from build123d import *
from OCP.BRepFilletAPI import BRepFilletAPI_MakeChamfer

# Parameters (mm, degrees)
SKETCH_47_W         = 56
SKETCH_47_H         = 48
EXTRUDE_4_DEPTH     = 43
CHAMFER_1_SIZE      = 10
CHAMFER_1_SIZE2     = 3.639702343
SHELL_1_T           = -3
CUT_EXTRUDE_3_REACH = 86.392
SKETCH_48_R         = 1
SKETCH_48_W         = 23.8
SKETCH_48_H         = 12.2
SKETCH_49_R         = 1.55
CUT_EXTRUDE_4_DEPTH = 71.263788682
CUT_EXTRUDE_5_REACH = 76.572
SKETCH_50_W         = 13
SKETCH_50_H         = 9
CUT_EXTRUDE_6_REACH = 76.572
SKETCH_51_W         = 10.719183514
SKETCH_51_H         = 21.879791556


with BuildPart() as part:
    # 草图47 → 凸台-拉伸4 (new body)
    with BuildSketch(Plane(origin=(0, 0, 0), x_dir=(1, 0, 0), z_dir=(0, 1, 0))):
        Rectangle(SKETCH_47_W, SKETCH_47_H)
    extrude(amount=EXTRUDE_4_DEPTH)

    # 倒角1: one chamfer whose edges measure the first distance from different faces: ONE call of the kernel's chamfer builder (chamfer() names one face for all edges)
    chamfer_1_edges_1 = [part.edges().sort_by_distance(p)[0] for p in [
        (28, 43, 0),
    ]]
    chamfer_1_side_1 = [part.faces().sort_by_distance(p)[0] for p in [
        (28, 21.5, 0),
    ]]
    chamfer_1_edges_2 = [part.edges().sort_by_distance(p)[0] for p in [
        (0, 43, -24),
    ]]
    chamfer_1_side_2 = [part.faces().sort_by_distance(p)[0] for p in [
        (0, 21.5, -24),
    ]]
    chamfer_1_edges_3 = [part.edges().sort_by_distance(p)[0] for p in [
        (-28, 43, 0),
    ]]
    chamfer_1_side_3 = [part.faces().sort_by_distance(p)[0] for p in [
        (-28, 21.5, 0),
    ]]
    chamfer_1_edges_4 = [part.edges().sort_by_distance(p)[0] for p in [
        (0, 43, 24),
    ]]
    chamfer_1_side_4 = [part.faces().sort_by_distance(p)[0] for p in [
        (0, 21.5, 24),
    ]]
    chamfer_1 = BRepFilletAPI_MakeChamfer(part.part.solid().wrapped)
    for e in chamfer_1_edges_1:
        chamfer_1.Add(CHAMFER_1_SIZE, CHAMFER_1_SIZE2, e.wrapped, chamfer_1_side_1[0].wrapped)  # the first distance lies on this face
    for e in chamfer_1_edges_2:
        chamfer_1.Add(CHAMFER_1_SIZE, CHAMFER_1_SIZE2, e.wrapped, chamfer_1_side_2[0].wrapped)  # the first distance lies on this face
    for e in chamfer_1_edges_3:
        chamfer_1.Add(CHAMFER_1_SIZE, CHAMFER_1_SIZE2, e.wrapped, chamfer_1_side_3[0].wrapped)  # the first distance lies on this face
    for e in chamfer_1_edges_4:
        chamfer_1.Add(CHAMFER_1_SIZE, CHAMFER_1_SIZE2, e.wrapped, chamfer_1_side_4[0].wrapped)  # the first distance lies on this face
    add(Compound.cast(chamfer_1.Shape()), mode=Mode.REPLACE)

    # 抽壳1
    shell_1_openings = [part.faces().sort_by_distance(p)[0] for p in [
        (0, 0, 0),
    ]]
    offset(amount=SHELL_1_T, openings=shell_1_openings, kind=Kind.INTERSECTION)

    # 草图48 → 切除-拉伸3 (cut, up to next)
    with BuildSketch(Plane(origin=(0, 43, -43), x_dir=(1, 0, 0), z_dir=(0, -1, 0)), mode=Mode.PRIVATE) as cut_extrude_3_sk1:
        with Locations(Location((-20.1, 43, 0), (0, 0, 90))):
            Circle(SKETCH_48_R)
    cut_extrude_3_tool1 = extrude(cut_extrude_3_sk1.sketch, amount=CUT_EXTRUDE_3_REACH, mode=Mode.PRIVATE) & part.part
    # 草图48 → 切除-拉伸3 (cut, up to next)
    with BuildSketch(Plane(origin=(0, 43, -43), x_dir=(1, 0, 0), z_dir=(0, -1, 0)), mode=Mode.PRIVATE) as cut_extrude_3_sk2:
        with Locations(Location((8.5, 43, 0), (0, 0, 90))):
            Circle(SKETCH_48_R)
    cut_extrude_3_tool2 = extrude(cut_extrude_3_sk2.sketch, amount=CUT_EXTRUDE_3_REACH, mode=Mode.PRIVATE) & part.part
    # 草图48 → 切除-拉伸3 (cut, up to next)
    with BuildSketch(Plane(origin=(0, 43, -43), x_dir=(1, 0, 0), z_dir=(0, -1, 0)), mode=Mode.PRIVATE) as cut_extrude_3_sk3:
        with Locations((-5.8, 43)):
            Rectangle(SKETCH_48_W, SKETCH_48_H)
    cut_extrude_3_tool3 = extrude(cut_extrude_3_sk3.sketch, amount=CUT_EXTRUDE_3_REACH, mode=Mode.PRIVATE) & part.part
    add(cut_extrude_3_tool1.solids().sort_by_distance((-20.1, 43, 0))[0], mode=Mode.SUBTRACT)
    add(cut_extrude_3_tool2.solids().sort_by_distance((8.5, 43, 0))[0], mode=Mode.SUBTRACT)
    add(cut_extrude_3_tool3.solids().sort_by_distance((-5.8, 43, 0))[0], mode=Mode.SUBTRACT)

    # 草图49 → 切除-拉伸4 (cut, through all)
    with BuildSketch(Plane(origin=(0, 0, -24), x_dir=(-1, 0, 0), z_dir=(0, 0, -1))):
        with Locations((0, 8)):
            Circle(SKETCH_49_R)
    extrude(amount=-CUT_EXTRUDE_4_DEPTH, mode=Mode.SUBTRACT)

    # 草图50 → 切除-拉伸5 (cut, up to next)
    with BuildSketch(Plane(origin=(28, 0, 0), x_dir=(0, 0, -1), z_dir=(1, 0, 0)), mode=Mode.PRIVATE) as cut_extrude_5_sk1:
        with Locations((0, 4.5)):
            Rectangle(SKETCH_50_W, SKETCH_50_H)
    cut_extrude_5_tool1 = extrude(cut_extrude_5_sk1.sketch, amount=-CUT_EXTRUDE_5_REACH, mode=Mode.PRIVATE) & part.part
    add(cut_extrude_5_tool1.solids().sort_by_distance((28, 4.5, 0))[0], mode=Mode.SUBTRACT)

    # 草图51 → 切除-拉伸6 (cut, up to next)
    with BuildSketch(Plane.ZY.offset(28), mode=Mode.PRIVATE) as cut_extrude_6_sk1:
        with Locations((0, 10.939895778)):
            Rectangle(SKETCH_51_W, SKETCH_51_H)
    cut_extrude_6_tool1 = extrude(cut_extrude_6_sk1.sketch, amount=-CUT_EXTRUDE_6_REACH, mode=Mode.PRIVATE) & part.part
    add(cut_extrude_6_tool1.solids().sort_by_distance((-28, 10.939896, 0))[0], mode=Mode.SUBTRACT)


solid = part.part
Part model, mm, in its own coordinate system. A direction names the side the tool comes from. Give positions to 0.01 mm unless a question says otherwise; leave off trailing zeros. Order: outer loops, then holes, each group sorted by start corner. A loop starts at its lowest first (then second) coordinate and runs counter-clockwise, first axis right, second up. Notation, with made-up numbers: (-21, 3) -> (38, 3) arc R13 ccw to (38, 13) -> close; hole circle Ø6 at (5.25, 22). An arc over 180 degrees is marked (long way). Use one line per item in the form item = value.
(1) Saw through at D-D (y = 21). Write the cut outline in (x, z), then the cut area to 3 significant figures.
Solution:
outline = (-28, -24) -> (28, -24) -> (28, 24) -> (-28, 24) -> (-28, 5.36) -> (-25, 5.36) -> (-25, 21) -> (25, 21) -> (25, -21) -> (-25, -21) -> (-25, -5.36) -> (-28, -5.36) -> close
area = 556 mm²
(2) Drill centre lines: line 1 (Z direction, x = -15, y = 14.5); line 2 (X direction, y = 41.7, z = 0); line 3 (X direction, y = 7, z = 17). Where is each one in solid material? Low to high. Write a range as from..to.
Solution:
line_1 = -24..-21, 21..24
line_2 = -24.83..-21.1, -19.1..-17.7, 6.1..7.5, 9.5..24.83
line_3 = -28..-25, 25..28
(3) Saw through at C-C (z = 0). Write the cut outline in (x, y), then the cut area to 3 significant figures.
Solution:
outline = (-28, 21.88) -> (-25, 21.88) -> (-25, 32.47) -> (-22.26, 40) -> (-21.1, 40) -> (-21.1, 43) -> (-24.36, 43) -> (-28, 33) -> close; (-19.1, 40) -> (-17.7, 40) -> (-17.7, 43) -> (-19.1, 43) -> close; (6.1, 40) -> (7.5, 40) -> (7.5, 43) -> (6.1, 43) -> close; (9.5, 40) -> (22.26, 40) -> (25, 32.47) -> (25, 9) -> (28, 9) -> (28, 33) -> (24.36, 43) -> (9.5, 43) -> close
area = 216 mm²
(4) Flat gauge pins, fed straight in: P1, Ø6, axis at y = 34, z = 9, coming from the -X side; P2, Ø4, axis at x = -12, y = 37.5, coming from the -Z side; P3, Ø0.9, axis at x = -3.5, y = 41.5, coming from the -Z side; P4, Ø1.9, axis at x = 0, y = 8, coming from the -Z side. Where does each tip first touch, or does it go through?
Solution:
P1 = -28
P2 = -23.09
P3 = -21.07
P4 = through
(5) Tool access for faces 5 (the face through (6.1, 42, 0)), 6 (the face through (0, 16, -21)), 7 (the face through (-27, 11, 5.36)): list every direction of +Z, -Z, +X, -X, +Y, -Y with a clear straight run to the whole face (end or side of a thin tool).
Solution:
face_5 = +Y, -Y
face_6 = -Y
face_7 = -X, -Y
(6) Pull direction X, two halves, no side cores. Call faces 1 (the face through (-0.715, 6.625, -22.521)), 2 (the face through (-27, 11, -5.36)), 3 (the face through (28, 16, 0)), 4 (the face through (-6, 42, 6.1)): +X half, -X half, draft (parallel to the pull), parting line (faces both ways), or undercut.
Solution:
face_1 = undercut
face_2 = draft
face_3 = +X half
face_4 = undercut
(7) Saw through at A-A (x = -20.1). Write the cut outline in (y, z), then the cut area to 3 significant figures.
Solution:
outline = (0, -24) -> (33, -24) -> (43, -20.36) -> (43, -1) -> (40, -1) -> (40, -18.26) -> (32.47, -21) -> (0, -21) -> close; (0, 21) -> (32.47, 21) -> (40, 18.26) -> (40, 1) -> (43, 1) -> (43, 20.36) -> (33, 24) -> (0, 24) -> close
area = 362 mm²
(8) Saw through at B-B (y = 8). Write the cut outline in (x, z).
Solution:
outline = (-28, -24) -> (-1.55, -24) -> (-1.55, -21) -> (-25, -21) -> (-25, -5.36) -> (-28, -5.36) -> close; (-28, 5.36) -> (-25, 5.36) -> (-25, 21) -> (-1.55, 21) -> (-1.55, 24) -> (-28, 24) -> close; (1.55, -24) -> (28, -24) -> (28, -6.5) -> (25, -6.5) -> (25, -21) -> (1.55, -21) -> close; (1.55, 21) -> (25, 21) -> (25, 6.5) -> (28, 6.5) -> (28, 24) -> (1.55, 24) -> close
